Solid Edge part; units mm, degrees
sketch "Sketch1" plane through (0, 0, 0) normal (0, 0, 1) x (1, 0, 0)
  circle A0 centre (0, 0) radius 41.05
  circle A1 centre (0, 0) radius 20.625
  circle A2 centre (164.42, 0) radius 23.37
  circle A3 centre (164.42, 0) radius 10
extrude "Protrusion1" add sketch "Sketch1" along normal blind 17.73
sketch "Sketch2" plane through (0, 0, 0) normal (0, 0, 1) x (1, 0, 0)
  line L0 (8.6399, 40.1305) -> (164.42, 23.37)
  line L1 (144.2869, 0) -> (164.42, 23.37)
  line L2 (164.42, -23.37) -> (144.2869, 0)
  line L3 (8.6399, -40.1305) -> (164.42, -23.37)
  line L4 (30.0194, 0) -> (8.6399, -40.1305)
  line L5 (8.6399, 40.1305) -> (30.0194, 0)
extrude "ExtrudedProtrusion_2" add sketch "Sketch2" along normal blind 12.7
sketch "Sketch3" plane through (0, 0, 0) normal (0, 0, 1) x (1, 0, 0)
  line L0 (-10.8125, 12.1278) -> (-5.0968, 15.4278)
  line L1 (-7.5968, 19.758) -> (-5.0968, 15.4278)
  line L2 (-13.3125, 16.458) -> (-7.5968, 19.758)
  line L3 (-10.8125, 12.1278) -> (-13.3125, 16.458)
  line L4 (-5.0968, -15.4278) -> (-7.5968, -19.758)
  line L5 (-7.5968, -19.758) -> (-13.3125, -16.458)
  line L6 (-13.3125, -16.458) -> (-10.8125, -12.1278)
  line L7 (-5.0968, -15.4278) -> (-10.8125, -12.1278)
  line L8 (15.9093, 3.3) -> (15.9093, -3.3)
  line L9 (20.9093, -3.3) -> (15.9093, -3.3)
  line L10 (20.9093, 3.3) -> (20.9093, -3.3)
  line L11 (15.9093, 3.3) -> (20.9093, 3.3)
extrude "Protrusion2" add sketch "Sketch3" along normal up to vertex (17.73 mm away)
The listing builds one solid part. Answer for the finished solid, in the listing's coordinates (mm). A direction names the side the tool comes from. Coordinates: 2 decimals unless noted, no trailing zeros. Write each loop counter-clockwise with the first axis right and the second up, starting at its lowest first coordinate (ties: lowest second). Pieces come first, ordered by that corner, then holes. Notation, with made-up numbers: (-30.75, -11.5) -> (-6.75, -11.5) arc R31 cw to (-6.75, 15.5) -> close; hole circle Ø9 at (59.5, 45.25). An arc over 180 degrees is marked (long way). Write each question's results on one line, items separated by ' | '. Start each with the question number.
1) A cutting plane is placed at C-C (x = 0). Determine the outline of the cut face in (y, z) (3 decimals), then the cut area to 3 significant figures.
2) A cutting plane is placed at B-B (y = 0). Determine the outline of the cut face in (x, z) (3 decimals), then the cut area to 3 significant figures.
3) Flat-ended cylindrical pins translate along their axes: pin 1 Ø6 at (x, z) = (88, 6.5) entering from +Y; pin 2 Ø10 at (x, z) = (36, 2.5) entering from -Y; pin 3 Ø3 at (x, z) = (27, 12.5) entering from +Y. Find the tip coordinate at first contact, or state that the pin passes through.
4) A tool of negligible diameter and unlimited length cuts with its end or side. For faces 5 (the cylindrical face through (186.71, -7.02, 10.71)), 6 (the flat face through (-7.915, -13.801, 8.741)), 7 (the flat face through (72, 1, 0)), from which of +Z, -Z, +X, -X, +Y, -Y can it reach the whole face along a straight path? Write none if from no direction.
5) For a pull along Y with two mould halves and no side action, classify faces 1 (the flat face through (-11.94, -14.08, 8.74)), 2 (the flat face through (18, 1, 17.73)), 3 (the cylindrical face through (-41, -2, 11)), 4 (the flat face through (85.439, -31.868, 6.261)) as +Y half, -Y half, draft (parallel to the pull), parting line (faces both ways), or undercut.
6) A cutting plane is placed at A-A (z = 4.75). Count the separate pieces of the cut face and the enclosed holes in it, then the cut area to 3 significant figures.
7) A cutting plane is placed at D-D (x = 147). Determine the outline of the cut face in (y, z).
8) Straight lines are drawn through the part: probe 1 along Y at (x, z) = (164.42, 11); probe 2 along Y at (x, z) = (18.5, 16.5); probe 3 along X at (y, z) = (14.5, 17). For each, find the intervals that lie inside material, in ascending order.
Values follow:
1) outline: (-41.05, 0) -> (-20.625, 0) -> (-20.625, 17.73) -> (-41.05, 17.73) -> close; (20.625, 0) -> (41.05, 0) -> (41.05, 17.73) -> (20.625, 17.73) -> close | area: 724 mm²
2) outline: (-41.05, 0) -> (-20.625, 0) -> (-20.625, 17.73) -> (-41.05, 17.73) -> close; (15.909, 0) -> (154.42, 0) -> (154.42, 17.73) -> (141.05, 17.73) -> (141.05, 12.7) -> (41.05, 12.7) -> (41.05, 17.73) -> (15.909, 17.73) -> close; (174.42, 0) -> (187.79, 0) -> (187.79, 17.73) -> (174.42, 17.73) -> close | area: 2,550 mm²
3) pin 1: y = 31.91 | pin 2: y = -37.72 | pin 3: y = 38.32
4) face 5: +Z | face 6: +Z, -Z | face 7: -Z, +X, -X, +Y, -Y
5) face 1: undercut | face 2: draft | face 3: parting line | face 4: -Y half
6) separate pieces: 1 | enclosed holes: 2 | area: 12,500 mm²
7) outline: (-25.24, 0) -> (25.24, 0) -> (25.24, 12.7) -> (15.58, 12.7) -> (15.58, 17.73) -> (-15.58, 17.73) -> (-15.58, 12.7) -> (-25.24, 12.7) -> close
8) probe 1: -23.37 to -10, 10 to 23.37 | probe 2: -36.64 to -9.12, -3.3 to 3.3, 9.12 to 36.64 | probe 3: -38.4 to -14.67, -12.18 to -6.7, 14.67 to 38.4, 146.09 to 182.75
